```python
from build123d import *

# Parameters (mm, degrees)
SKETCH1_W                   = 68.58
SKETCH1_H                   = 22.86
EXTRUDE1_DEPTH              = 9.652
SKETCH4_W                   = 68.58
SKETCH4_H                   = 3.81
EXTRUDE3_DEPTH              = 12.192
F_5_16_CLEARANCE_HOLE1_D    = 8.2042
SKETCH3_W                   = 68.58
SKETCH3_H                   = 9.144
EXTRUDE2_DEPTH              = 1.016
SKETCH6_W                   = 68.58
SKETCH6_H                   = 1.3462
CUT_EXTRUDE2_DEPTH          = 10.652
F_1_4_20_TAPPED_HOLE1_D     = 5.1054
F_1_4_20_TAPPED_HOLE1_DEPTH = 19.05
F_1_4_20_TAPPED_HOLE1_TIP   = 1.533816902


with BuildPart() as part:
    # Sketch1 → Extrude1 (new body)
    with BuildSketch(Plane(origin=(0, 0, 0), x_dir=(1, 0, 0), z_dir=(0, 1, 0))):
        Rectangle(SKETCH1_W, SKETCH1_H)
    extrude(amount=EXTRUDE1_DEPTH)

    # Sketch4 → Extrude3 (add)
    with BuildSketch(Plane(origin=(0, 9.652, 0), x_dir=(1, 0, 0), z_dir=(0, 1, 0))):
        with Locations((0, -11.8872)):
            Rectangle(SKETCH4_W, SKETCH4_H)
    extrude(amount=-EXTRUDE3_DEPTH)

    # 5/16 Clearance Hole1 (through all)
    with Locations(Plane(origin=(-22.86, 0, -0.0508), x_dir=(0, 0, -1), z_dir=(0, -1, 0))):
        with Locations((0, 0), (0, 45.72), (0, 22.86)):
            Hole(F_5_16_CLEARANCE_HOLE1_D / 2)

    # Sketch3 → Extrude2 (cut)
    with BuildSketch(Plane.XZ):
        with Locations((0, -0.0508)):
            Rectangle(SKETCH3_W, SKETCH3_H)
    extrude(amount=-EXTRUDE2_DEPTH, mode=Mode.SUBTRACT)

    # Sketch6 → Cut-Extrude2 (cut, through all)
    with BuildSketch(Plane.XZ):
        with Locations((0, -10.7569)):
            Rectangle(SKETCH6_W, SKETCH6_H)
    extrude(amount=-CUT_EXTRUDE2_DEPTH, mode=Mode.SUBTRACT)

    # 1/4-20 Tapped Hole1
    with Locations(Plane(origin=(0, 9.652, 0), x_dir=(-1, 0, 0), z_dir=(0, 1, 0))):
        with Locations((11.43, -5.1308), (11.43, 7.5692), (-11.43, 7.5692), (-11.43, -5.1308)):
            Hole(F_1_4_20_TAPPED_HOLE1_D / 2, depth=F_1_4_20_TAPPED_HOLE1_DEPTH)
            with Locations((0, 0, -(F_1_4_20_TAPPED_HOLE1_DEPTH + F_1_4_20_TAPPED_HOLE1_TIP / 2))):  # 118° drill point
                Cone(0, F_1_4_20_TAPPED_HOLE1_D / 2, F_1_4_20_TAPPED_HOLE1_TIP, mode=Mode.SUBTRACT)


solid = part.part
```
Input: part model. Units: mm. Frame: model coordinates. A direction names the side the tool comes from. Coordinates: 2 decimals unless noted, no trailing zeros. Loops run counter-clockwise (first coordinate to the right, second up) from the corner with the lowest first, then second, coordinate; pieces in that order, holes last. Notation, with made-up numbers: (74.5, 63.25) - (116.5, 63.25) arc R25 ccw to (116.5, 91.25) - close; hole circle Ø5 at (-18.75, 56.25). An arc over 180 degrees is marked (long way). Answer in a Markdown table with one row per item.
(1) Cut plane D-D on z = -6.75. Output: boundary loops of the cut face in (x, y), plus the area to 3 significant figures.
Model answer:
| item | result |
|---|---|
| outline | (-34.29, 0) - (-13.4, 0) - (-13.4, 9.65) - (-34.29, 9.65) - close; (-9.46, 0) - (9.46, 0) - (9.46, 9.65) - (-9.46, 9.65) - close; (13.4, 0) - (34.29, 0) - (34.29, 9.65) - (13.4, 9.65) - close |
| area | 586 mm² |
(2) Cut plane B-B on x = -11.43. Output: boundary loops of the cut face in (y, z), plus the area to 3 significant figures.
Model answer:
| item | result |
|---|---|
| outline | (-2.54, 10.12) - (9.65, 10.12) - (9.65, 13.79) - (-2.54, 13.79) - close; (0, -10.08) - (9.65, -10.08) - (9.65, -7.68) - (0, -7.68) - close; (0, 4.52) - (1.02, 4.52) - (1.02, -2.58) - (9.65, -2.58) - (9.65, 5.02) - (0, 5.02) - close |
| area | 134 mm² |
(3) Cut plane A-A on x = 0. Output: boundary loops of the cut face in (y, z), plus the area to 3 significant figures.
Model answer:
| item | result |
|---|---|
| outline | (-2.54, 9.98) - (0, 9.98) - (0, 4.52) - (1.02, 4.52) - (1.02, 4.05) - (9.65, 4.05) - (9.65, 13.79) - (-2.54, 13.79) - close; (0, -10.08) - (9.65, -10.08) - (9.65, -4.15) - (1.02, -4.15) - (1.02, -4.62) - (0, -4.62) - close |
| area | 160 mm² |
(4) Cut plane C-C on y = -1. Output: boundary loops of the cut face in (x, z).
Model answer:
| item | result |
|---|---|
| outline | (-34.29, 9.98) - (-12.26, 9.98) arc R2.55 cw to (-10.6, 9.98) - (10.6, 9.98) arc R2.55 cw to (12.26, 9.98) - (34.29, 9.98) - (34.29, 13.79) - (-34.29, 13.79) - close |
(5) Set-up query: faces 1 (the face through (7, 1.016, 0)), 2 (the face through (0, 5, -10.084)), 3 (the face through (-23, -1, 9.982)). Return all of +Z, -Z, +X, -X, +Y, -Y with unobstructed straight access to the full face (end or side cutting, diameter ignored); none if empty.
Model answer:
| item | result |
|---|---|
| face 1 | +X, -X, -Y |
| face 2 | -Z, +X, -X, +Y, -Y |
| face 3 | -Z, +X, -X, -Y |
(6) Pin query (flat end, axial travel): P1, Ø2.5, axis at x = -13.5, z = 2, coming from the -Y side; P2, Ø6, axis at x = -20, z = -5.5, coming from the -Y side; P3, Ø1.3, axis at x = -5, y = -1, coming from the -Z side. Return the tip coordinate at first contact, or that it passes through.
Model answer:
| item | result |
|---|---|
| P1 | stops at y = 1.02 |
| P2 | stops at y = 0 |
| P3 | stops at z = 9.98 |
(7) Material intervals for L1, parallel to X at y = 0.25, z = 7.75; L2, parallel to Z at x = 11.43, y = 4.25; L3, parallel to X at y = 1.5, z = 0.25, sorted ascending. Write a range as from..to.
Model answer:
| item | result |
|---|---|
| L1 | x = -34.29..-13.98, -8.88..8.88, 13.98..34.29 |
| L2 | z = -10.08..-7.68, -2.58..5.02, 10.12..13.79 |
| L3 | x = -34.29..-26.95, -18.77..-4.09, 4.09..18.77, 26.95..34.29 |
(8) Mould query, pull axis X, two halves, no side actions, for faces 4 (the face through (-11.983, 4.758, -7.623)), 5 (the face through (34.29, 5, 2)), 6 (the face through (0, 4, 13.792)). Classes: pulls with the +X half, pulls with the -X half, needs draft (parallel to the pull), parting line crosses it, or undercut.
Model answer:
| item | result |
|---|---|
| face 4 | undercut |
| face 5 | pulls with the +X half |
| face 6 | needs draft |
